Can you work these out from the drawing? Everything is in mm from the part's minimum corner. Give positions to 0.01 mm unless a question says otherwise; leave off trailing zeros. Order: outer loops, then holes, each group sorted by start corner. A loop starts at its lowest first (then second) coordinate and runs counter-clockwise, first axis right, second up. Notation, with made-up numbers: (-17, 33.25) - (8, 33.25) arc R21 ccw to (8, 57.25) - close; hole circle Ø11 at (78.25, -37). An arc over 180 degrees is marked (long way). One line per question, with ' | ' between items.
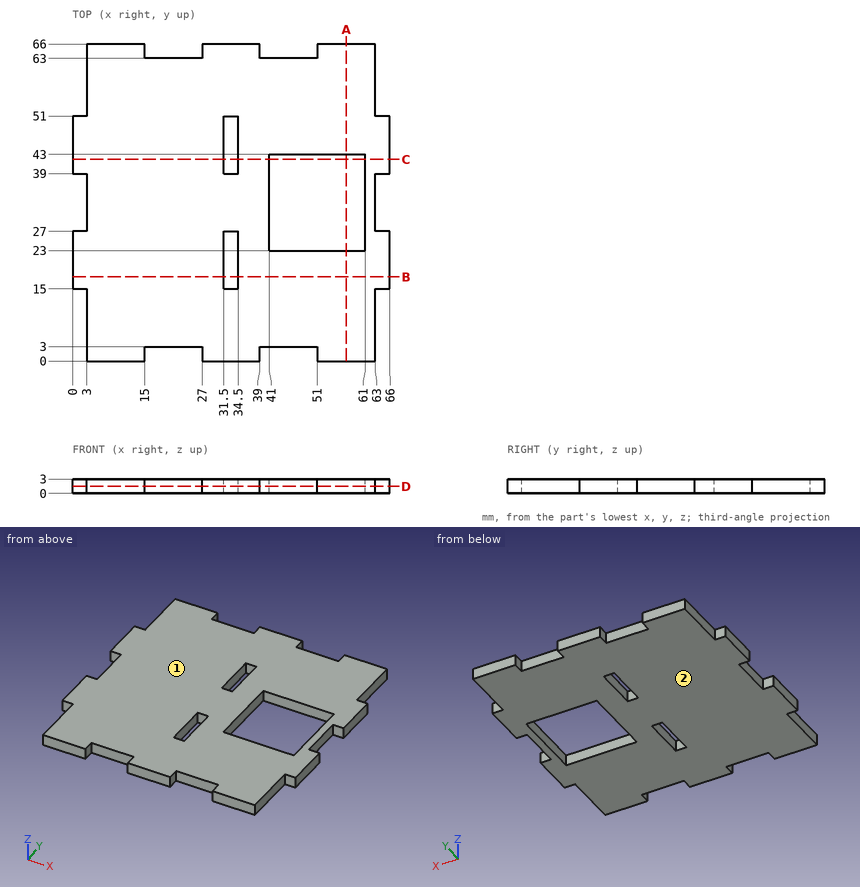
1) I want a section at D-D (z = 1.45). State how many separate pieces and enclosed holes the cut face has, plus the area to 3 significant figures.
Model answer:
separate pieces: 1 | enclosed holes: 3 | area: 3,490 mm2
2) I'm going to push flat-ended pins straight in: P1, Ø1.5, axis at y = 6, z = 2, coming from the -X side; P2, Ø8, axis at x = 46, y = 53.5, coming from the -Z side; P3, Ø1.5, axis at y = 29.5, z = 0.5, coming from the +X side; P4, Ø0.9, axis at x = 23, z = 2, coming from the +Y side. Where does each tip first touch, or does it pass through?
Model answer:
P1: stops at x = 3 | P2: stops at z = 0 | P3: stops at x = 63 | P4: stops at y = 63
3) I want a section at C-C (y = 42). List the corners of the cut face in (x, z) for me, plus the area to 3 significant figures.
Model answer:
outline: (0, 0) - (31.5, 0) - (31.5, 3) - (0, 3) - close; (34.5, 0) - (41, 0) - (41, 3) - (34.5, 3) - close; (61, 0) - (66, 0) - (66, 3) - (61, 3) - close | area: 129 mm2
4) I want a section at B-B (y = 17.5). List the corners of the cut face in (x, z) for me, plus the area to 3 significant figures.
Model answer:
outline: (0, 0) - (31.5, 0) - (31.5, 3) - (0, 3) - close; (34.5, 0) - (66, 0) - (66, 3) - (34.5, 3) - close | area: 189 mm2
5) Thinking about a two-plate mould opening in Z: for the marked faces 1 and 2, which applies, +Z half, -Z half, draft (parallel to the pull), parting line (faces both ways), or undercut?
Model answer:
face 1: +Z half | face 2: -Z half
6) I want a section at A-A (x = 57). List the corners of the cut face in (y, z) for me.
Model answer:
outline: (0, 0) - (23, 0) - (23, 3) - (0, 3) - close; (43, 0) - (66, 0) - (66, 3) - (43, 3) - close
7) Please list where these lines run through material, in increasing order: L1, parallel to X at y = 24, z = 1.65; L2, parallel to X at y = 20.5, z = 1.35; L3, parallel to Y at x = 51.5, z = 0.45.
Model answer:
L1: x = 0 to 31.5, 34.5 to 41, 61 to 66 | L2: x = 0 to 31.5, 34.5 to 66 | L3: y = 0 to 23, 43 to 66
